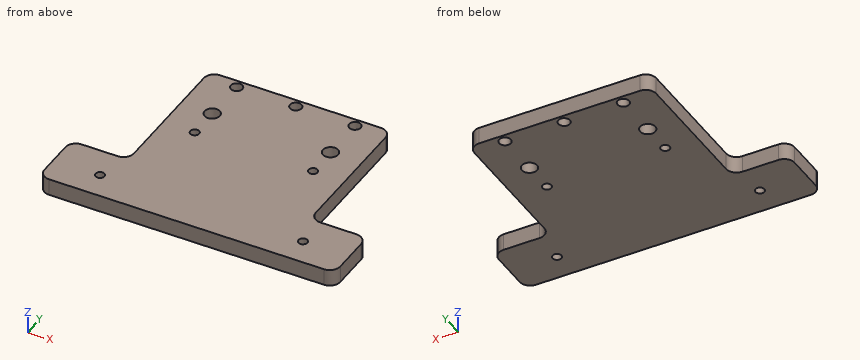
from build123d import *

# Parameters (mm, degrees)
PAD_DEPTH     = 8
SKETCH033_R   = 2.1
HOLE007_DEPTH = 25
SKETCH035_R   = 3.6
HOLE009_DEPTH = 25
SKETCH036_R   = 2.1
HOLE010_DEPTH = 25
SKETCH051_R   = 2.75
HOLE018_DEPTH = 25


with BuildPart() as part:
    # Sketch → Pad (new body)
    with BuildSketch(Plane.XY):
        with BuildLine():
            Line((-38, -31.56), (38, -31.56))
            ThreePointArc((43, -36.56), (41.535534, -33.024466), (38, -31.56))
            Line((43, -36.56), (43, -96.544143))
            ThreePointArc((43, -96.544143), (44.464466, -100.079677), (48, -101.544143))
            Line((48, -101.544143), (65, -101.544143))
            ThreePointArc((70, -106.544143), (68.535534, -103.008609), (65, -101.544143))
            Line((70, -106.544143), (70, -124.41))
            ThreePointArc((65, -129.41), (68.535534, -127.945534), (70, -124.41))
            Line((65, -129.41), (-65, -129.41))
            ThreePointArc((-70, -124.41), (-68.535534, -127.945534), (-65, -129.41))
            Line((-70, -124.41), (-70, -106.544143))
            ThreePointArc((-65, -101.544143), (-68.535534, -103.008609), (-70, -106.544143))
            Line((-65, -101.544143), (-48, -101.544143))
            ThreePointArc((-48, -101.544143), (-44.464466, -100.079677), (-43, -96.544143))
            Line((-43, -96.544143), (-43, -36.56))
            ThreePointArc((-38, -31.56), (-41.535534, -33.024466), (-43, -36.56))
        make_face()
    extrude(amount=PAD_DEPTH)

    # Sketch033 (on Face17 of Pad) → Hole007 (cut)
    with BuildSketch(Plane(origin=(0, 0, 0), x_dir=(1, 0, 0), z_dir=(0, 0, -1))):
        with Locations((-48, 116.56)):
            Circle(SKETCH033_R)
        with Locations((48, 116.56)):
            Circle(SKETCH033_R)
    extrude(amount=-HOLE007_DEPTH, mode=Mode.SUBTRACT)

    # Sketch035 (on Face17 of Pad) → Hole009 (cut)
    with BuildSketch(Plane(origin=(0, 0, 0), x_dir=(1, 0, 0), z_dir=(0, 0, -1))):
        with Locations((-28, 56.56)):
            Circle(SKETCH035_R)
        with Locations((28, 56.56)):
            Circle(SKETCH035_R)
    extrude(amount=-HOLE009_DEPTH, mode=Mode.SUBTRACT)

    # Sketch036 (on Hole) → Hole010 (cut)
    with BuildSketch(Plane.XY):
        with Locations((-28, -71.57)):
            Circle(SKETCH036_R)
        with Locations((28, -71.57)):
            Circle(SKETCH036_R)
    extrude(amount=HOLE010_DEPTH, mode=Mode.SUBTRACT)

    # Sketch051 (on Hole) → Hole018 (cut)
    with BuildSketch(Plane.XY):
        with Locations((-28, -35.56)):
            Circle(SKETCH051_R)
        with Locations((0, -35.56)):
            Circle(SKETCH051_R)
        with Locations((28, -35.56)):
            Circle(SKETCH051_R)
    extrude(amount=HOLE018_DEPTH, mode=Mode.SUBTRACT)


solid = part.part
For this review, take the finished solid that the model builds, in its own axes (mm). Give positions to 0.01 mm unless a question says otherwise; leave off trailing zeros. Loops run counter-clockwise (first coordinate to the right, second up) from the corner with the lowest first, then second, coordinate; pieces in that order, holes last. Notation, with made-up numbers: M 9,34.25 L 63,34.25 A22 ccw 63,60.25 Z; hole C 30.25,73 d6. An arc over 180 degrees is marked long. Put each result on its own line as item: value. Start each with the question number.
(1) Add section A-A, the plane y = -71.57. Write out the cut boundary in (x, z), then the cut area to 3 significant figures.
(2) Add section B-B, the plane z = 5.75. Give the number of separate pieces and of enclosed holes in the cut face, then the cut area to 3 significant figures.
(3) Add section D-D, the plane y = -56.56. Write out the cut boundary in (x, z).
(4) Add section C-C, the plane x = 28. Write out the cut boundary in (y, z).
(5) Wall thickness on L1, parallel to Y at x = -28, z = 3.75; L2, parallel to X at y = -116.56, z = 5.5; L3, parallel to Y at x = -48, z = 3.25: over which ranges is each line inside the solid? List them lowest first.
(6) For pin 1 (4 mm diameter, centred on y = -67.5, z = 3, fed in from -X); pin 2 (3 mm diameter, centred on y = -65, z = 5, fed in from +X); pin 3 (4 mm diameter, centred on x = -58, z = 4, fed in from +Y), all flat-tipped, find the tip position at first contact; note any pin that passes through.
Result:
1. outline: M -43,0 L -30.1,0 L -30.1,8 L -43,8 Z; M -25.9,0 L 25.9,0 L 25.9,8 L -25.9,8 Z; M 30.1,0 L 43,0 L 43,8 L 30.1,8 Z
1. area: 621 mm^2
2. separate pieces: 1
2. enclosed holes: 9
2. area: 9,690 mm^2
3. outline: M -43,0 L -31.6,0 L -31.6,8 L -43,8 Z; M -24.4,0 L 24.4,0 L 24.4,8 L -24.4,8 Z; M 31.6,0 L 43,0 L 43,8 L 31.6,8 Z
4. outline: M -129.41,0 L -73.67,0 L -73.67,8 L -129.41,8 Z; M -69.47,0 L -60.16,0 L -60.16,8 L -69.47,8 Z; M -52.96,0 L -38.31,0 L -38.31,8 L -52.96,8 Z; M -32.81,0 L -31.56,0 L -31.56,8 L -32.81,8 Z
5. L1: y = -129.41 to -73.67, -69.47 to -60.16, -52.96 to -38.31, -32.81 to -31.56
5. L2: x = -70 to -50.1, -45.9 to 45.9, 50.1 to 70
5. L3: y = -129.41 to -118.66, -114.46 to -101.54
6. pin 1: stops at x = -43
6. pin 2: stops at x = 43
6. pin 3: stops at y = -101.54
